Read the model definition and answer for the solid it produces. Units are mm, in the model's axes. Face numbers are marked on the shaded views. Coordinates: 2 decimals unless noted, no trailing zeros. Write each loop counter-clockwise with the first axis right and the second up, starting at its lowest first coordinate (ties: lowest second). Pieces come first, ordered by that corner, then holes. Notation, with made-up numbers: M 73,18.5 L 97,18.5 A20 cw 97,42.5 Z; hole C 81,76.5 d8. An arc over 180 degrees is marked long. Write item = value, one per line.
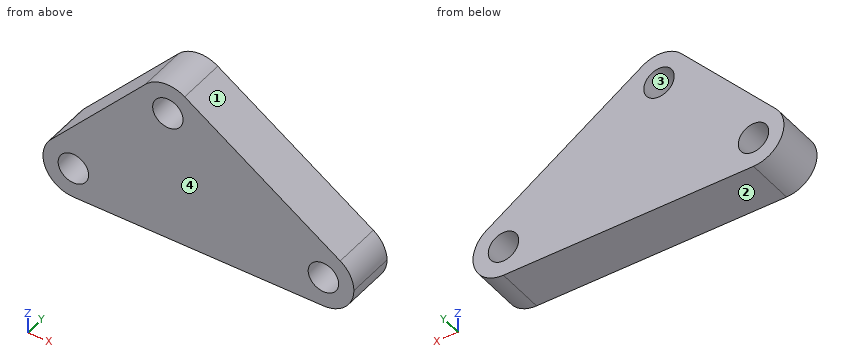
from build123d import *

# Parameters (mm, degrees)
F1_DEPTH = 12.7
F2_R     = 4
F3_DEPTH = 12.7


with BuildPart() as f1:
    # F0 (on Front) → F1 (new body)
    with BuildSketch(Plane.XZ):
        with BuildLine():
            Line((-35.8775282965, 24.0157592565), (-21.8738068975, 39.259964286))
            ThreePointArc((-21.8738068975, 39.259964286), (-24.4545549996, 44.812447626), (-22.3532208609, 50.5635107317))
            Line((-22.3532208609, 50.5635107317), (-47.1810747422, 23.536345293))
            ThreePointArc((-47.1810747422, 23.536345293), (-41.6285914022, 26.1170933952), (-35.8775282965, 24.0157592565))
        make_face()
        with BuildLine():
            Line((-21.8738068975, 39.259964286), (-16.4617406563, 45.1514444906))
            Line((-16.4617406563, 45.1514444906), (-9.7887372084, 40.7388460516))
            ThreePointArc((-9.7887372084, 40.7388460516), (-8.8006693349, 42.8475377633), (-8.4617406563, 45.1514444906))
            ThreePointArc((-8.4617406563, 45.1514444906), (-9.4154371037, 48.939531903), (-12.0491422174, 51.8244479385))
            ThreePointArc((-12.0491422174, 51.8244479385), (-17.4334728618, 53.0922087183), (-22.3532208609, 50.5635107317))
            ThreePointArc((-22.3532208609, 50.5635107317), (-24.4545549996, 44.812447626), (-21.8738068975, 39.259964286))
        make_face()
        with BuildLine():
            ThreePointArc((-9.7887372084, 40.7388460516), (-15.4900084509, 37.2106802628), (-21.8738068975, 39.259964286))
            Line((-21.8738068975, 39.259964286), (-35.8775282965, 24.0157592565))
            ThreePointArc((-35.8775282965, 24.0157592565), (-33.9650969463, 21.3416902838), (-33.2895945376, 18.1242790519))
            Line((-33.2895945376, 18.1242790519), (16.4104054624, 18.1242790519))
            ThreePointArc((16.4104054624, 18.1242790519), (16.749334141, 20.4281857792), (17.7374020144, 22.5368774909))
            Line((17.7374020144, 22.5368774909), (-9.7887372084, 40.7388460516))
        make_face()
        with BuildLine():
            Line((-9.7887372084, 40.7388460516), (-16.4617406563, 45.1514444906))
            Line((-16.4617406563, 45.1514444906), (-21.8738068975, 39.259964286))
            ThreePointArc((-21.8738068975, 39.259964286), (-15.4900084509, 37.2106802628), (-9.7887372084, 40.7388460516))
        make_face()
        with BuildLine():
            ThreePointArc((-8.4617406563, 45.1514444906), (-8.8006693349, 42.8475377633), (-9.7887372084, 40.7388460516))
            Line((-9.7887372084, 40.7388460516), (17.7374020144, 22.5368774909))
            ThreePointArc((17.7374020144, 22.5368774909), (22.8120577523, 25.9629833197), (28.8230039014, 24.7972824999))
            Line((28.8230039014, 24.7972824999), (-12.0491422174, 51.8244479385))
            ThreePointArc((-12.0491422174, 51.8244479385), (-9.4154371037, 48.939531903), (-8.4617406563, 45.1514444906))
        make_face()
        with BuildLine():
            ThreePointArc((28.8230039014, 24.7972824999), (22.8120577523, 25.9629833197), (17.7374020144, 22.5368774909))
            Line((17.7374020144, 22.5368774909), (24.4104054624, 18.1242790519))
            Line((24.4104054624, 18.1242790519), (16.4104054624, 18.1242790519))
            ThreePointArc((16.4104054624, 18.1242790519), (18.7535512129, 12.4674248024), (24.4104054624, 10.1242790519))
            ThreePointArc((24.4104054624, 10.1242790519), (30.0672597119, 12.4674248024), (32.4104054624, 18.1242790519))
            ThreePointArc((32.4104054624, 18.1242790519), (31.456709015, 21.9123664643), (28.8230039014, 24.7972824999))
        make_face()
        with BuildLine():
            Line((24.4104054624, 18.1242790519), (17.7374020144, 22.5368774909))
            ThreePointArc((17.7374020144, 22.5368774909), (16.749334141, 20.4281857792), (16.4104054624, 18.1242790519))
            Line((16.4104054624, 18.1242790519), (24.4104054624, 18.1242790519))
        make_face()
        with BuildLine():
            Line((16.4104054624, 18.1242790519), (-33.2895945376, 18.1242790519))
            ThreePointArc((-33.2895945376, 18.1242790519), (-35.6327402881, 12.4674248024), (-41.2895945376, 10.1242790519))
            Line((-41.2895945376, 10.1242790519), (24.4104054624, 10.1242790519))
            ThreePointArc((24.4104054624, 10.1242790519), (18.7535512129, 12.4674248024), (16.4104054624, 18.1242790519))
        make_face()
        with BuildLine():
            Line((-41.2895945376, 18.1242790519), (-35.8775282965, 24.0157592565))
            ThreePointArc((-35.8775282965, 24.0157592565), (-41.6285914022, 26.1170933952), (-47.1810747422, 23.536345293))
            ThreePointArc((-47.1810747422, 23.536345293), (-48.6140921289, 14.90686782), (-41.2895945376, 10.1242790519))
            ThreePointArc((-41.2895945376, 10.1242790519), (-35.6327402881, 12.4674248024), (-33.2895945376, 18.1242790519))
            Line((-33.2895945376, 18.1242790519), (-41.2895945376, 18.1242790519))
        make_face()
        with BuildLine():
            ThreePointArc((-33.2895945376, 18.1242790519), (-33.9650969463, 21.3416902838), (-35.8775282965, 24.0157592565))
            Line((-35.8775282965, 24.0157592565), (-41.2895945376, 18.1242790519))
            Line((-41.2895945376, 18.1242790519), (-33.2895945376, 18.1242790519))
        make_face()
    extrude(amount=F1_DEPTH)

    # F2 (on face) → F3 (cut, through all)
    with BuildSketch(Plane.XZ.offset(12.7)):
        with Locations((-16.4617406563, 45.1514444906)):
            Circle(F2_R)
        with Locations((-41.2895945376, 18.1242790519)):
            Circle(F2_R)
        with Locations((24.4104054624, 18.1242790519)):
            Circle(F2_R)
    extrude(amount=-F3_DEPTH, mode=Mode.SUBTRACT)


solid = f1.part
Item 1: Find section D-D (x = 11). Determine the outline of the cut face in (y, z), and give its area (3 significant figures).
Worked answers:
outline = M -12.7,10.12 L 0,10.12 L 0,36.58 L -12.7,36.58 Z
area = 336 mm²
Item 2: Find section B-B (y = -10.5). Determine the outline of the cut face in (x, z), and give its area (3 significant figures).
Worked answers:
outline = M -47.18,23.54 A8 ccw -41.29,10.12 L 24.41,10.12 A8 ccw 28.82,24.8 L -12.05,51.82 A8 ccw -22.35,50.56 Z; hole C -41.29,18.12 d8; hole C -16.46,45.15 d8; hole C 24.41,18.12 d8
area = 2,150 mm²
Item 3: Find section A-A (x = 21.5). Determine the outline of the cut face in (y, z), and give its area (3 significant figures).
Worked answers:
outline = M -12.7,10.12 L 0,10.12 L 0,15.38 L -12.7,15.38 Z; M -12.7,20.87 L 0,20.87 L 0,29.64 L -12.7,29.64 Z
area = 178 mm²
Item 4: For a pull along Z with two mould halves and no side action, classify the marked faces 1, 2, 3 and 4 as released by +Z, released by -Z, zero draft, split by the parting line, or undercut.
Worked answers:
face_1 = released by +Z
face_2 = released by -Z
face_3 = undercut
face_4 = zero draft
Item 5: Flat-ended cylindrical pins translate along their axes: pin 1 (4 mm diameter, centred on y = -6, z = 36.5, fed in from -X); pin 2 (1 mm diameter, centred on y = -1.5, z = 47.5, fed in from -X); pin 3 (3 mm diameter, centred on y = -4, z = 28, fed in from +X). Find the tip coordinate at first contact, or state that the pin passes through.
Worked answers:
pin_1 = -37.11
pin_2 = -25.63
pin_3 = 26.25
Item 6: Consider line 1 along Z through (x, y) = (-43.5, -11); line 2 along X through (y, z) = (-12, 45); line 3 along X through (y, z) = (-12, 41.5). Determine where each line is inside the solid, lowest interval first. Write a range as from..to.
Worked answers:
line_1 = 10.44..14.79, 21.46..27.54
line_2 = -27.46..-20.46, -12.46..-1.73
line_3 = -30.68..-18.09, -14.83..3.56
Item 7: Find section C-C (z = 47). Determine the outline of the cut face in (x, y), and give its area (3 significant figures).
Worked answers:
outline = M -25.63,-12.7 L -20.01,-12.7 L -20.01,0 L -25.63,0 Z; M -12.91,-12.7 L -4.75,-12.7 L -4.75,0 L -12.91,0 Z
area = 175 mm²
